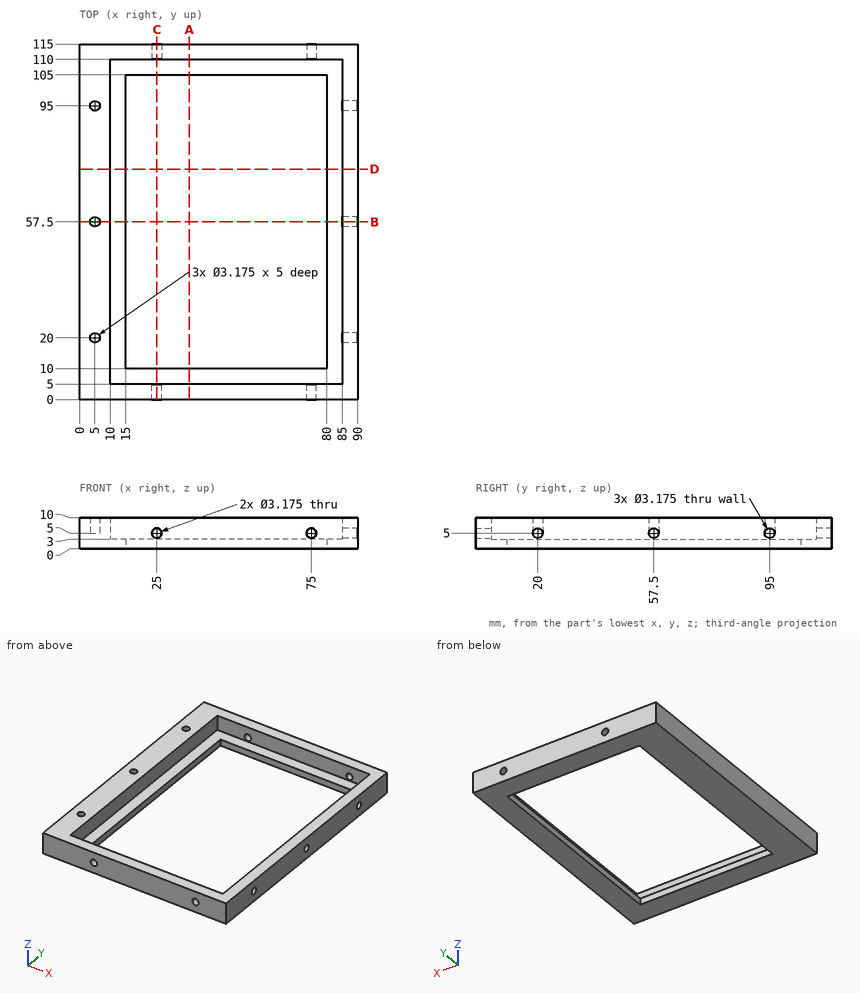
Here's the drawing with two shaded views (mm, measured from the low corner). I have some questions. Coordinates: 2 decimals unless noted, no trailing zeros. Write each loop counter-clockwise with the first axis right and the second up, starting at its lowest first coordinate (ties: lowest second). Pieces come first, ordered by that corner, then holes. Notation, with made-up numbers: M -40,-12.75 L 18,-12.75 A31 ccw 18,16.25 Z; hole C -40,-37.5 d2. An arc over 180 degrees is marked long. Write item = value, one per line. Start each with the question number.
Q1. If I drill on L1, parallel to X at y = 112.85, z = 5; L2, parallel to X at y = 95, z = 8.7; L3, parallel to Y at x = 73, z = 3.5, over which ranges is the centre line in solid material (lowest first)? Write a range as [from, to].
Q2. I'm going to push flat-ended pins straight in: pin 1 (4 mm diameter, centred on x = 75, z = 5, fed in from +Y); pin 2 (1.9 mm diameter, centred on x = 5, y = 20, fed in from +Z). Where does each tip first touch, or does it pass through?
Q3. If we section it at D-D, the plane y = 74.5: Write out the boundary of the cut face in (x, z), then the cut area to 3 significant figures.
Q4. If we section it at C-C, the plane x = 25: Write out the boundary of the cut face in (y, z), then the cut area to 4 significant figures.
Q5. If we section it at B-B, the plane y = 57.5: Write out the boundary of the cut face in (x, z), then the cut area to 3 significant figures.
Q6. If we section it at A-A, the plane x = 35.5: Write out the boundary of the cut face in (y, z), then the cut area to 3 significant figures.
Check sheet entries:
q1.L1 = [0, 23.41], [26.59, 73.41], [76.59, 90]
q1.L2 = [0, 3.41], [6.59, 10], [85, 90]
q1.L3 = [0, 5], [110, 115]
q2.pin_1 = 115
q2.pin_2 = 5
q3.outline = M 0,0 L 15,0 L 15,3 L 10,3 L 10,10 L 0,10 Z; M 80,0 L 90,0 L 90,10 L 85,10 L 85,3 L 80,3 Z
q3.area = 180 mm²
q4.outline = M 0,0 L 10,0 L 10,3 L 5,3 L 5,3.41 L 0,3.41 Z; M 0,6.59 L 5,6.59 L 5,10 L 0,10 Z; M 105,0 L 115,0 L 115,3.41 L 110,3.41 L 110,3 L 105,3 Z; M 110,6.59 L 115,6.59 L 115,10 L 110,10 Z
q4.area = 98.25 mm²
q5.outline = M 0,0 L 15,0 L 15,3 L 10,3 L 10,10 L 6.59,10 L 6.59,5 L 3.41,5 L 3.41,10 L 0,10 Z; M 80,0 L 90,0 L 90,3.41 L 85,3.41 L 85,3 L 80,3 Z; M 85,6.59 L 90,6.59 L 90,10 L 85,10 Z
q5.area = 148 mm²
q6.outline = M 0,0 L 10,0 L 10,3 L 5,3 L 5,10 L 0,10 Z; M 105,0 L 115,0 L 115,10 L 110,10 L 110,3 L 105,3 Z
q6.area = 130 mm²
